Autodesk Inventor part; units mm, degrees
ref_plane "Work Plane1" through (0, 0, -25) normal (0, 0, 1) x (1, 0, 0)
ref_plane "Work Plane5" through (72, 5.9974, -20) normal (0, 1, 0) x (1, 0, 0)
ref_plane "YZ Plane" through (0, 0, 0) normal (1, 0, 0) x (0, 1, 0)
ref_plane "Work Plane1" through (0, 0, -25) normal (0, 0, 1) x (1, 0, 0)
sketch "Sketch4" plane through (0, 0, -25) normal (0, 0, 1) x (1, 0, 0)
  line L0 (70, -4.0026) -> (70, 3.9974)
  line L1 (72, 5.9974) -> (90, 5.9974)
  line L2 (90, 5.9974) -> (90, 3.4974)
  line L3 (90, 3.4974) -> (77, 3.4974)
  line L4 (75, 1.4974) -> (75, 0.4974)
  line L5 (77, -1.5026) -> (90, -1.5026)
  line L6 (90, -1.5026) -> (90, -4.0026)
  line L7 (90, -4.0026) -> (70, -4.0026)
  arc A0 (72, 5.9974) -> (70, 3.9974) centre (72, 3.9974) ccw
  arc A1 (77, 3.4974) -> (75, 1.4974) centre (77, 1.4974) ccw
  arc A2 (75, 0.4974) -> (77, -1.5026) centre (77, 0.4974) ccw
  line L8 (70, 0) -> (70, -3)
  line L9 (55, -4.0026) -> (55, -2.0026)
  line L10 (55, -2.0026) -> (68, -2.0026)
  line L11 (68, -2.0026) -> (68, 0.9974)
  line L12 (68, 0.9974) -> (55, 0.9974)
  line L13 (55, -4.0026) -> (70, -4.0026)
  line L14 (55, 0.9974) -> (55, 2.9974)
  line L15 (55, 2.9974) -> (70, 2.9974)
  point P0 (0, 0)
  dimension "d66" = 5
  dimension "d67" = 2.5
  dimension "d68" = 2.5
  dimension "d69" = 20
  dimension "d70" = 15
  dimension "d71" = 2
  dimension "d111" = 2
  dimension "d112" = 2
  dimension "d113" = 3
  dimension "d115" = 2
  dimension "d116" = 15
  dimension "d117" = 15
ref_plane "Work Plane5" through (72, 5.9974, -20) normal (0, 1, 0) x (1, 0, 0)
sketch "Sketch5" plane through (72, 5.9974, -20) normal (0, 1, 0) x (1, 0, 0)
  line L0 (18, 10) -> (18, 0)
  line L1 (0, 10) -> (18, 10)
  point P0 (-72, -20)
  point P1 (15, 5)
  dimension "d86" = 3
  dimension "d87" = 5
hole "Hole1" [suppressed]
extrude "Extrusion5" add sketch "Sketch4" along normal mid plane 10
hole "Hole2" at (87, 5.9974, -25) direction (0, -1, 0) diameter 3 end through all
sketch "Sketch8" plane through (55, 2.9974, -20) normal (0, 1, 0) x (1, 0, 0)
  line L0 (0, 10) -> (15, 10)
  line L1 (0, 10) -> (0, 0)
  point P0 (-55, -20)
  point P1 (5, 5)
  dimension "d127" = 5
  dimension "d128" = 5
hole "Hole3" at (60, 2.9974, -25) direction (0, -1, 0) diameter 3 end through all
thread "Thread1"
thread "Thread2"
thread "Thread3"
thread "Thread4"
properties part number "base_plate" material "PC/ABS Plastic"
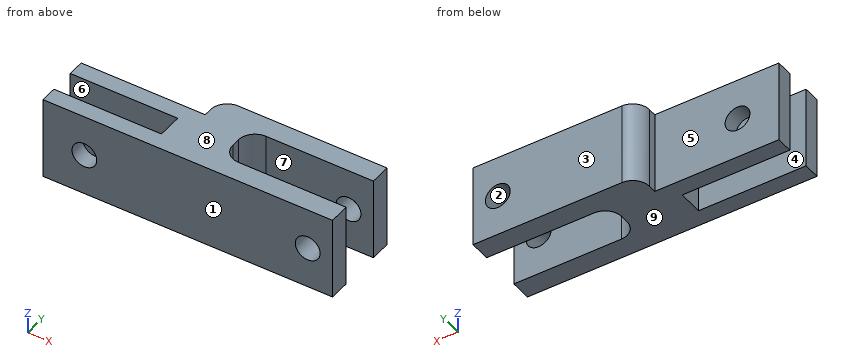
Design review of the part built by this model. Coordinates are the model's own, in mm. Face numbers are marked on the shaded views. A direction names the side the tool comes from. Coordinates: 2 decimals unless noted, no trailing zeros. Write each loop counter-clockwise with the first axis right and the second up, starting at its lowest first coordinate (ties: lowest second). Pieces come first, ordered by that corner, then holes. Notation, with made-up numbers: M -38,33 L 3,33 A27 cw 3,60 Z; hole C -23,15.5 d5. An arc over 180 degrees is marked long. Answer as a JSON object with one key per item and string values.
Item 1: Add section C-C, the plane y = -2.5. Give the boundary of the cut face in (x, z), and give its area (3 significant figures).
Outcome:
{"outline": "M 55,-30 L 90,-30 L 90,-20 L 55,-20 Z; hole C 60,-25 d3; hole C 87,-25 d3", "area": "336 mm²"}
Item 2: Add section A-A, the plane z = -25. State how many separate pieces and enclosed holes the cut face has, and give its area (3 significant figures).
Outcome:
{"separate pieces": "5", "enclosed holes": "0", "area": "165 mm²"}
Item 3: Insertion check: pin 1 Ø3 at (x, z) = (62, -25.5) entering from +Y; pin 2 Ø0.8 at (y, z) = (3.5, -24.5) entering from -X; pin 3 Ø0.9 at (y, z) = (-0.5, -27) entering from -X. Each pin has a flat end and moves straight along its axis. Give the tip position at first contact, or say it passes through.
Outcome:
{"pin 1": "y = 3", "pin 2": "x = 70", "pin 3": "x = 68"}
Item 4: Wall thickness on probe 1 along Y at (x, z) = (82.5, -25); probe 2 along Z at (x, y) = (87, -1.95); probe 3 along Y at (x, z) = (62.5, -25.25): over which ranges is each line inside the solid? List them lowest first.
Outcome:
{"probe 1": "-4 to -1.5, 3.5 to 6", "probe 2": "-30 to -26.5, -23.5 to -20", "probe 3": "-4 to -2, 1 to 3"}
Item 5: Add section D-D, the plane z = -27.25. Give the boundary of the cut face in (x, y), and give its area (3 significant figures).
Outcome:
{"outline": "M 55,-4 L 90,-4 L 90,-1.5 L 77,-1.5 A2 cw 75,0.5 L 75,1.5 A2 cw 77,3.5 L 90,3.5 L 90,6 L 72,6 A2 ccw 70,4 L 70,3 L 55,3 L 55,1 L 68,1 L 68,-2 L 55,-2 Z", "area": "192 mm²"}
Item 6: Add section B-B, the plane x = 87. Give the boundary of the cut face in (y, z).
Outcome:
{"outline": "M -4,-30 L -1.5,-30 L -1.5,-26.5 L -4,-26.5 Z; M -4,-23.5 L -1.5,-23.5 L -1.5,-20 L -4,-20 Z; M 3.5,-30 L 6,-30 L 6,-26.5 L 3.5,-26.5 Z; M 3.5,-23.5 L 6,-23.5 L 6,-20 L 3.5,-20 Z"}
Item 7: Machinability: for the marked faces 5, 6, 7, 8 and 9, which of the approach directions +Z, -Z, +X, -X, +Y, -Y give a long, thin tool a straight path to every point of the face, cutting with its end or side? Answer none if there is none.
Outcome:
{"face 5": "+Z, -Z, -X, +Y", "face 6": "+Z, -Z, -X", "face 7": "+Z, -Z, +X", "face 8": "+Z, +X, -X, +Y, -Y", "face 9": "-Z, +X, -X, +Y, -Y"}
Item 8: Draft analysis for pull direction Y (two halves, no side actions). For the marked faces 1, 2, 3 and 4, state which applies: pulls with the +Y half, pulls with the -Y half, needs draft (parallel to the pull), parting line crosses it, or undercut.
Outcome:
{"face 1": "pulls with the -Y half", "face 2": "needs draft", "face 3": "pulls with the +Y half", "face 4": "undercut"}
